from build123d import *

# Parameters (mm, degrees)
SKETCH_W      = 198
SKETCH_H      = 112.5
PAD_DEPTH     = 3
FILLET_R      = 5
SKETCH001_R   = 1.5
SKETCH001_R_2 = 10
POCKET_DEPTH  = 3.001
FILLET001_R   = 20


with BuildPart() as part:
    # Sketch → Pad (new body)
    with BuildSketch(Plane.XY):
        Rectangle(SKETCH_W, SKETCH_H)
    extrude(amount=PAD_DEPTH)

    # Fillet
    fillet_edges = [part.edges().sort_by_distance(p)[0] for p in [
        (-99, 56.25, 1.5),
        (99, 56.25, 1.5),
    ]]
    fillet(fillet_edges, radius=FILLET_R)

    # Sketch001 (on Face5 of Fillet) → Pocket (cut, through all)
    with BuildSketch(Plane.XY.offset(3)):
        with Locations((-93, 46.25)):
            Circle(SKETCH001_R)
        with Locations((-93, -43.92)):
            Circle(SKETCH001_R)
        with Locations((93, 46.25)):
            Circle(SKETCH001_R)
        with Locations((93, -43.92)):
            Circle(SKETCH001_R)
        with Locations((-23.15, 46.25)):
            Circle(SKETCH001_R)
        with Locations((23.15, 46.25)):
            Circle(SKETCH001_R)
        with Locations((0, 41.25)):
            Circle(SKETCH001_R_2)
        with BuildLine():
            Line((-13.5, -32.25), (13.5, -32.25))
            ThreePointArc((15, -33.75), (14.56066, -32.68934), (13.5, -32.25))
            Line((15, -33.75), (15, -56.25))
            Line((15, -56.25), (-15, -56.25))
            Line((-15, -56.25), (-15, -33.75))
            ThreePointArc((-13.5, -32.25), (-14.56066, -32.68934), (-15, -33.75))
        make_face()
    extrude(amount=-POCKET_DEPTH, mode=Mode.SUBTRACT)

    # Fillet001
    fillet001_edges = [part.edges().sort_by_distance(p)[0] for p in [
        (-15, -56.25, 1.5),
        (15, -56.25, 1.5),
    ]]
    fillet(fillet001_edges, radius=FILLET001_R)


solid = part.part
Read the model definition and answer for the solid it produces. Units are mm, in the model's axes. A direction names the side the tool comes from. Coordinates: 2 decimals unless noted, no trailing zeros. Loops run counter-clockwise (first coordinate to the right, second up) from the corner with the lowest first, then second, coordinate; pieces in that order, holes last.
Q1. The part is cut by section A-A on x = 0. Write down the section's boundary in (y, z).
Q2. Consider probe 1 along Y at (x, z) = (93, 1.3); probe 2 along X at (y, z) = (-35, 2.6); probe 3 along Y at (x, z) = (3, 2.8). Determine where each line is inside the solid, lowest interval first.
Q3. The part is cut by section B-B on z = 1.1. Write down the section's boundary in (x, y).
Q4. The mould has two halves that part along X. Classify faces 3 (the face through (-1, 1, 3)), 4 (the face through (-97.57, 54.75, 1.52)), 5 (the face through (-21.014, -50.547, 1.479)): +X half, -X half, draft (parallel to the pull), parting line (faces both ways), or undercut.
Q5. Each of these flat-tipped pins is pushed along its axis until it touches: pin 1 Ø2.5 at (x, y) = (23.15, 46.25) entering from -Z; pin 2 Ø0.9 at (x, z) = (1.5, 2) entering from -Y. Where does it stop, or does it pass through?
Q6. The part is cut by section C-C on y = 39. Write down the section's boundary in (x, z), and give its area (3 significant figures).
Q7. Which of the six approach directions +Z, -Z, +X, -X, +Y, -Y give full straight-line access (tool end or side, diameter ignored) to faces 1 (the face through (21.014, -50.547, 1.479)), 2 (the face through (97.57, 54.75, 1.52))?
Results below:
1. outline: (-32.25, 0) - (31.25, 0) - (31.25, 3) - (-32.25, 3) - close; (51.25, 0) - (56.25, 0) - (56.25, 3) - (51.25, 3) - close
2. probe 1: y = -56.25 to -45.42, -42.42 to 44.75, 47.75 to 56.25
2. probe 2: x = -99 to -15, 15 to 99
2. probe 3: y = -32.25 to 31.71, 50.79 to 56.25
3. outline: (-99, -56.25) - (-35, -56.25) arc R20 ccw to (-15, -36.25) - (-15, -33.75) arc R1.5 cw to (-13.5, -32.25) - (13.5, -32.25) arc R1.5 cw to (15, -33.75) - (15, -36.25) arc R20 ccw to (35, -56.25) - (99, -56.25) - (99, 51.25) arc R5 ccw to (94, 56.25) - (-94, 56.25) arc R5 ccw to (-99, 51.25) - close; hole circle Ø3 at (-93, -43.92); hole circle Ø3 at (-93, 46.25); hole circle Ø3 at (-23.15, 46.25); hole circle Ø20 at (0, 41.25); hole circle Ø3 at (23.15, 46.25); hole circle Ø3 at (93, -43.92); hole circle Ø3 at (93, 46.25)
4. face 3: draft
4. face 4: -X half
4. face 5: undercut
5. pin 1: passes through
5. pin 2: stops at y = -32.25
6. outline: (-99, 0) - (-9.74, 0) - (-9.74, 3) - (-99, 3) - close; (9.74, 0) - (99, 0) - (99, 3) - (9.74, 3) - close
6. area: 536 mm2
7. face 1: +Z, -Z, -Y
7. face 2: +Z, -Z, +X, +Y
